from build123d import *

# Parameters (mm, degrees)
SKETCH1_R           = 2.475
SKETCH1_R_2         = 1.5
BOSS_EXTRUDE1_DEPTH = 5
BOSS_EXTRUDE2_START = 5
SKETCH1_2_R         = 2.475
SKETCH1_2_R_2       = 1.5
BOSS_EXTRUDE2_DEPTH = 5
SKETCH2_R           = 4
SKETCH2_R_2         = 2.075
BOSS_EXTRUDE3_DEPTH = 2
FILLET1_R           = 0.5


with BuildPart() as part:
    # Sketch1 → Boss-Extrude1 (new body)
    with BuildSketch(Plane(origin=(0, 0, 0), x_dir=(1, 0, 0), z_dir=(0, 1, 0))):
        Circle(SKETCH1_R)
        Circle(SKETCH1_R_2, mode=Mode.SUBTRACT)
    extrude(amount=BOSS_EXTRUDE1_DEPTH)

    # Sketch1<2> → Boss-Extrude2 (add)
    with BuildSketch(Plane(origin=(0, 0, 0), x_dir=(1, 0, 0), z_dir=(0, 1, 0)).offset(BOSS_EXTRUDE2_START)):
        Circle(SKETCH1_2_R)
        Circle(SKETCH1_2_R_2, mode=Mode.SUBTRACT)
        Circle(SKETCH1_2_R_2)
    extrude(amount=BOSS_EXTRUDE2_DEPTH)

    # Sketch2 → Boss-Extrude3 (add)
    with BuildSketch(Plane(origin=(0, 10, 0), x_dir=(1, 0, 0), z_dir=(0, 1, 0))):
        Circle(SKETCH2_R)
        Circle(SKETCH2_R_2, mode=Mode.SUBTRACT)
    extrude(amount=BOSS_EXTRUDE3_DEPTH)

    # Fillet1
    fillet1_edges = [part.edges().sort_by_distance(p)[0] for p in [
        (-2.475, 10, 0),
        (-2.075, 10, 0),
    ]]
    fillet(fillet1_edges, radius=FILLET1_R)


solid = part.part
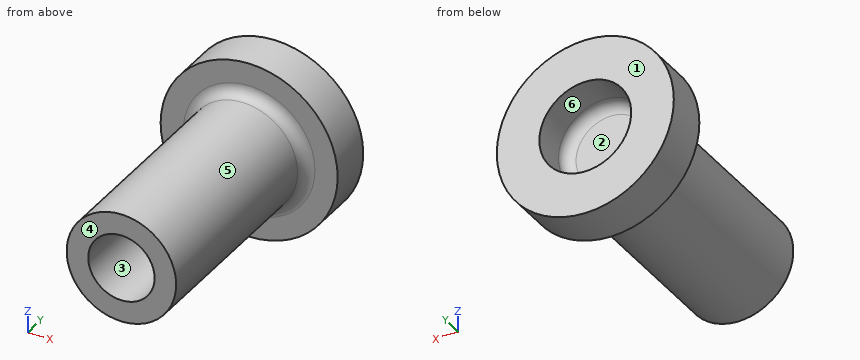
The listing builds one solid part. Answer for the finished solid, in the listing's coordinates (mm). Face numbers are marked on the shaded views. A direction names the side the tool comes from. Round coordinates to 2 decimals unless told otherwise and drop trailing zeros. Write each loop counter-clockwise with the first axis right and the second up, starting at its lowest first coordinate (ties: lowest second). Pieces come first, ordered by that corner, then holes. Notation, with made-up numbers: M -29,67.25 L -1,67.25 A21 ccw -1,74.25 Z; hole C 53.5,27 d8. An arc over 180 degrees is marked long. Write each question's results on one line, items separated by ' | '. Start each with the question number.
Item 1: Flat-ended cylindrical pins translate along their axes: pin 1 Ø2.5 at (x, z) = (-0.5, 0) entering from +Y; pin 2 Ø3 at (y, z) = (6, -0.5) entering from +X (3 decimals); pin 3 Ø1 at (y, z) = (6, 0.5) entering from -X (3 decimals). Find the tip coordinate at first contact, or state that the pin passes through.
Item 2: A cutting plane is placed at C-C on y = 2. Write down the section's boundary in (x, z) (3 decimals).
Item 3: For the marked faces 1, 2 and 3, determine the directions among +Z, -Z, +X, -X, +Y, -Y from which every point of the face is accessible in a straight line to the end or side of a thin tool.
Item 4: A cutting plane is placed at B-B on x = 0. Write down the section's boundary in (y, z) (3 decimals), and give its area (3 significant figures).
Item 5: For a pull along X with two mould halves and no side action, classify the marked faces 4, 5 and 6 as pulls with the +X half, pulls with the -X half, needs draft (parallel to the pull), parting line crosses it, or undercut.
Item 6: A cutting plane is placed at A-A on z = 0. Write down the section's boundary in (x, y) (3 decimals), and give its area (3 significant figures).
Item 7: Straight lines are drawn through the part: L1, parallel to X at y = 11.2, z = 0 (3 decimals); L2, parallel to Z at x = 0, y = 1.5 (3 decimals). For each, find the intervals that lie inside material, in ascending order. Write a range as [from, to].
Item 8: A cutting plane is placed at D-D on y = 10.75. Write down the section's boundary in (x, z) (3 decimals), and give its area (3 significant figures).
Check sheet entries:
1) pin 1: y = 10.03 | pin 2: x = 2.475 | pin 3: x = -2.475
2) outline: C 0,0 d4.95; hole C 0,0 d3
3) face 1: +Z, -Z, +X, -X, +Y | face 2: +Y | face 3: -Y
4) outline: M 0,-2.475 L 9.5,-2.475 A0.5 cw 10,-2.975 L 10,-4 L 12,-4 L 12,-2.075 L 10.5,-2.075 A0.5 cw 10,-1.575 L 10,1.575 A0.5 cw 10.5,2.075 L 12,2.075 L 12,4 L 10,4 L 10,2.975 A0.5 cw 9.5,2.475 L 0,2.475 L 0,1.5 L 5,1.5 L 5,-1.5 L 0,-1.5 Z | area: 42.4 mm²
5) face 4: needs draft | face 5: parting line crosses it | face 6: undercut
6) outline: M -4,10 L -2.975,10 A0.5 cw -2.475,9.5 L -2.475,0 L -1.5,0 L -1.5,5 L 1.5,5 L 1.5,0 L 2.475,0 L 2.475,9.5 A0.5 cw 2.975,10 L 4,10 L 4,12 L 2.075,12 L 2.075,10.5 A0.5 cw 1.575,10 L -1.575,10 A0.5 cw -2.075,10.5 L -2.075,12 L -4,12 Z | area: 42.4 mm²
7) L1: [-4, -2.075], [2.075, 4] | L2: [-2.475, -1.5], [1.5, 2.475]
8) outline: C 0,0 d8; hole C 0,0 d4.15 | area: 36.7 mm²
